from build123d import *

# Parameters (mm, degrees)
BOSS_EXTRUDE1_DEPTH = 38
SKETCH3_R           = 1.4
CUT_EXTRUDE2_DEPTH  = 8
SKETCH4_W           = 20.5
SKETCH4_H           = 41
CUT_EXTRUDE4_DEPTH  = 14
SKETCH7_R           = 1.4
CUT_EXTRUDE6_DEPTH  = 8
FILLET1_R           = 1.5
FILLET2_R           = 1.5


with BuildPart() as part:
    # Sketch1 → Boss-Extrude1 (new body)
    with BuildSketch(Plane.XY):
        Polygon((0, 0), (90, 0), (90, 71), (77, 71), (77, 10), (0, 10), align=None)
    extrude(amount=BOSS_EXTRUDE1_DEPTH)

    # Sketch3 → Cut-Extrude2 (cut)
    with BuildSketch(Plane.XZ):
        with Locations((23.6, 19)):
            Circle(SKETCH3_R)
        with Locations((34.1, 29.5)):
            Circle(SKETCH3_R)
        with Locations((44.6, 19)):
            Circle(SKETCH3_R)
        with Locations((34.1, 8.5)):
            Circle(SKETCH3_R)
    extrude(amount=-CUT_EXTRUDE2_DEPTH, mode=Mode.SUBTRACT)

    # Sketch4 → Cut-Extrude4 (cut, through all)
    with BuildSketch(Plane.ZY.offset(-77)):
        with Locations((18.854791971, 40.5)):
            Rectangle(SKETCH4_W, SKETCH4_H)
    extrude(amount=-CUT_EXTRUDE4_DEPTH, mode=Mode.SUBTRACT)

    # Sketch7 → Cut-Extrude6 (cut)
    with BuildSketch(Plane.ZY.offset(-77)):
        with Locations((13.906550577, 65.016024352)):
            Circle(SKETCH7_R)
        with Locations((23.806550577, 65.016024352)):
            Circle(SKETCH7_R)
        with Locations((13.906550577, 16.416024352)):
            Circle(SKETCH7_R)
        with Locations((23.806550577, 16.416024352)):
            Circle(SKETCH7_R)
    extrude(amount=-CUT_EXTRUDE6_DEPTH, mode=Mode.SUBTRACT)

    # Fillet1
    fillet1_edges = [part.edges().sort_by_distance(p)[0] for p in [
        (83.5, 20, 8.604791971),
        (83.5, 61, 8.604791971),
        (83.5, 61, 29.104791971),
        (83.5, 20, 29.104791971),
    ]]
    fillet(fillet1_edges, radius=FILLET1_R)

    # Fillet2
    fillet2_edges = [part.edges().sort_by_distance(p)[0] for p in [
        (77, 10, 19),
        (90, 0, 19),
        (83.5, 71, 38),
        (0, 5, 38),
        (83.5, 71, 0),
        (0, 5, 0),
    ]]
    fillet(fillet2_edges, radius=FILLET2_R)


solid = part.part
Geometry check sheet. Reference: the model listing, model coordinates, mm. A direction names the side the tool comes from. Round coordinates to 2 decimals unless told otherwise and drop trailing zeros. Write each loop counter-clockwise with the first axis right and the second up, starting at its lowest first coordinate (ties: lowest second). Pieces come first, ordered by that corner, then holes. Notation, with made-up numbers: (49, 86.5) - (83, 86.5) arc R23 ccw to (83, 97.5) - close; hole circle Ø2 at (29, -8). An arc over 180 degrees is marked (long way). One line per item, written item: value.
1. Cross-section at C-C on x = 44.6. Record the boundary of the cut face in (y, z).
The answers:
outline: (0, 0) - (10, 0) - (10, 38) - (0, 38) - (0, 20.4) - (8, 20.4) - (8, 17.6) - (0, 17.6) - close
2. Scan lines: L1, parallel to Y at x = 53.5, z = 9.5; L2, parallel to X at y = 39, z = 30; L3, parallel to Y at x = 79, z = 10.5. Record each from-to range of solid material in increasing order.
The answers:
L1: y = 0 to 10
L2: x = 77 to 90
L3: y = 0 to 20, 61 to 71
3. Cross-section at A-A on z = 19. Record the boundary of the cut face in (x, y).
The answers:
outline: (0, 0) - (22.2, 0) - (22.2, 8) - (25, 8) - (25, 0) - (43.2, 0) - (43.2, 8) - (46, 8) - (46, 0) - (88.5, 0) arc R1.5 ccw to (90, 1.5) - (90, 20) - (77, 20) - (77, 11.5) arc R1.5 cw to (75.5, 10) - (0, 10) - close; (77, 61) - (90, 61) - (90, 71) - (77, 71) - close
4. Mould release check, pull along Z, two halves, no side actions. Record for faces 5 (the face through (34, 8, 30)), 6 (the face through (59, 9, 0)), 7 (the face through (44, 0, 15)): released by +Z, released by -Z, zero draft, split by the parting line, or undercut.
The answers:
face 5: undercut
face 6: released by -Z
face 7: zero draft
5. Set-up check for faces 1 (the face through (85, 65, 24)), 2 (the face through (77, 42, 31)), 3 (the face through (34.85, 3.94, 30.68)), 4 (the face through (83, 61, 19)): record each of +Z, -Z, +X, -X, +Y, -Y from which the full face is reachable in a straight line by a thin tool's end or side.
The answers:
face 1: -X
face 2: +Z, -Z, -X, +Y
face 3: -Y
face 4: +X, -X
6. Cross-section at B-B on y = 35. Record the boundary of the cut face in (x, z), and give its area (4 significant figures).
The answers:
outline: (77, 0) - (90, 0) - (90, 8.6) - (77, 8.6) - close; (77, 29.1) - (90, 29.1) - (90, 38) - (77, 38) - close
area: 227.5 mm^2
7. Cross-section at D-D on z = 33. Record the boundary of the cut face in (x, y), and give its area (3 significant figures).
The answers:
outline: (0, 0) - (88.5, 0) arc R1.5 ccw to (90, 1.5) - (90, 71) - (77, 71) - (77, 11.5) arc R1.5 cw to (75.5, 10) - (0, 10) - close
area: 1,690 mm^2
8. Depth check by flat-ended pin: pin 1 Ø2.5 at (y, z) = (16.42, 13.91) entering from -X; pin 2 Ø2.5 at (x, z) = (34.1, 29.5) entering from +Y; pin 3 Ø1.4 at (x, z) = (23.5, 19) entering from -Y; pin 4 Ø12 at (x, y) = (74, 45) entering from +Z. Enter the tip coordinate at first touch or a pass-through.
The answers:
pin 1: stops at x = 85
pin 2: stops at y = 10
pin 3: stops at y = 8
pin 4: stops at z = 38
